For this review, use the dimensioned drawing (mm, ordinates from the lowest corner) and the shaded views. A direction names the side the tool comes from. Round coordinates to 2 decimals unless told otherwise and drop trailing zeros. Loops run counter-clockwise (first coordinate to the right, second up) from the corner with the lowest first, then second, coordinate; pieces in that order, holes last. Notation, with made-up numbers: (21, 67.25) -> (61, 67.25) arc R24 ccw to (61, 80.25) -> close; hole circle Ø5 at (13, 51). An arc over 180 degrees is marked (long way). Write each question's results on one line, items separated by ' | '.
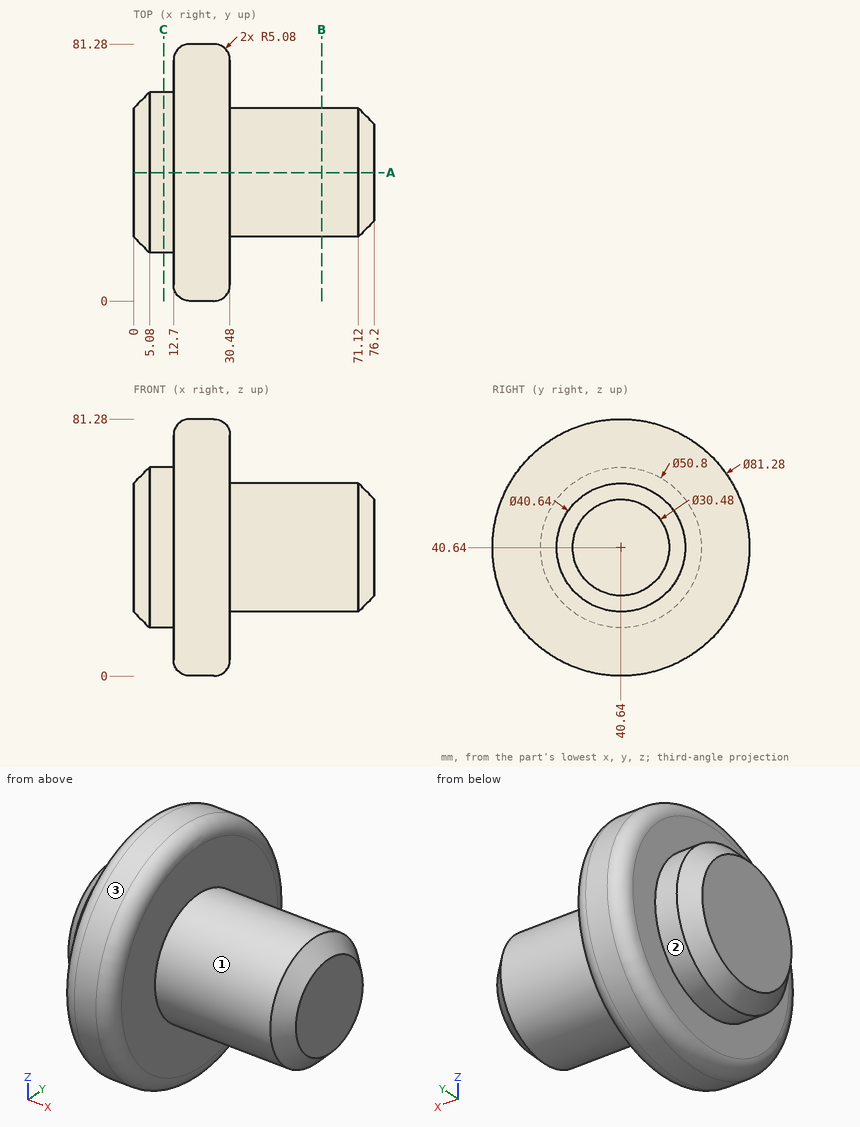
1. Consider section B-B (x = 59.5). State the section outline as (y, z) points, plus the area to 3 significant figures.
Values found:
outline: circle Ø40.64 at (40.64, 40.64) | area: 1,300 mm2
2. Consider section C-C (x = 9.5). State the section outline as (y, z) points, plus the area to 3 significant figures.
Values found:
outline: circle Ø50.8 at (40.64, 40.64) | area: 2,030 mm2
3. For pin 1 (8 mm diameter, centred on x = 12.5, z = 54, fed in from +Y); pin 2 (2 mm diameter, centred on y = 16, z = 52.5, fed in from -X); pin 3 (1 mm diameter, centred on x = 30, y = 19, fed in from -Z), all flat-tipped, find the tip position at first contact; note any pin that passes through.
Values found:
pin 1: stops at y = 79.32 | pin 2: stops at x = 12.7 | pin 3: stops at z = 8.66
4. Tool access review of the marked faces 1, 2 and 3: name each direction out of +Z, -Z, +X, -X, +Y, -Y from which nothing blocks a thin tool from reaching the whole face with its end or side.
Values found:
face 1: +X | face 2: -X | face 3: +X, -X
5. To check wall thickness, follow probe 1 along X at (y, z) = (53, 9); probe 2 along Y at (x, z) = (10.5, 41); probe 3 along Y at (x, z) = (58.5, 36.5). State the ranges of each line that lie inside material, in increasing order.
Values found:
probe 1: x = 12.7 to 30.48 | probe 2: y = 15.24 to 66.04 | probe 3: y = 20.75 to 60.53
6. Consider section A-A (y = 40.64). State the section outline as (x, z) points.
Values found:
outline: (0, 20.32) -> (5.08, 15.24) -> (12.7, 15.24) -> (12.7, 5.08) arc R5.08 ccw to (17.78, 0) -> (25.4, 0) arc R5.08 ccw to (30.48, 5.08) -> (30.48, 20.32) -> (71.12, 20.32) -> (76.2, 25.4) -> (76.2, 55.88) -> (71.12, 60.96) -> (30.48, 60.96) -> (30.48, 76.2) arc R5.08 ccw to (25.4, 81.28) -> (17.78, 81.28) arc R5.08 ccw to (12.7, 76.2) -> (12.7, 66.04) -> (5.08, 66.04) -> (0, 60.96) -> close
